from build123d import *

# Parameters (mm, degrees)
SKETCH1_R           = 2.75
BOSS_EXTRUDE1_DEPTH = 3
BOSS_EXTRUDE2_DEPTH = 3
CUT_EXTRUDE3_DEPTH  = 3.981121947


with BuildPart() as part:
    # Sketch1 → Boss-Extrude1 (new body)
    with BuildSketch(Plane(origin=(0, 0, 0), x_dir=(1, 0, 0), z_dir=(0, 1, 0))):
        with Locations(Location((0, 0, 0), (0, 0, 270))):
            Circle(SKETCH1_R)
    extrude(amount=BOSS_EXTRUDE1_DEPTH)

    # Sketch2 → Boss-Extrude2 (add)
    with BuildSketch(Plane(origin=(0, 0, 0), x_dir=(1, 0, 0), z_dir=(0, 1, 0))):
        Polygon((0.721687836, 1.25), (-0.721687836, 1.25), (-1.443375673, 0), (-0.721687836, -1.25), (0.721687836, -1.25), (1.443375673, 0), align=None)
    extrude(amount=BOSS_EXTRUDE2_DEPTH)

    # Sketch2_2 → Cut-Extrude3 (cut)
    with BuildSketch(Plane(origin=(0, 0, 0), x_dir=(1, 0, 0), z_dir=(0, 1, 0))):
        Polygon((0.721687836, 1.25), (-0.721687836, 1.25), (-1.443375673, 0), (-0.721687836, -1.25), (0.721687836, -1.25), (1.443375673, 0), align=None)
    extrude(amount=CUT_EXTRUDE3_DEPTH, mode=Mode.SUBTRACT)


solid = part.part
Build history of the part. All positions in model axes, mm. A direction names the side the tool comes from. Coordinates: 2 decimals unless noted, no trailing zeros. Order: outer loops, then holes, each group sorted by start corner. A loop starts at its lowest first (then second) coordinate and runs counter-clockwise, first axis right, second up. Notation, with made-up numbers: (66, 64) - (101, 64) arc R25 cw to (101, 93) - close; hole circle Ø3 at (14, 78). An arc over 180 degrees is marked (long way). Put each result on its own line as item: value.
1. Drop flat-ended pins along their axis: P1, Ø1.5, axis at y = 1.5, z = -1, coming from the -X side; P2, Ø1, axis at x = 1.5, z = 1.5, coming from the -Y side; P3, Ø0.7, axis at x = 0.5, y = 2, coming from the +Z side; P4, Ø1, axis at x = 2, y = 1.5, coming from the +Z side. Give the stop position or say it passes through.
Answer sheet:
P1: stops at x = -2.74
P2: stops at y = 0
P3: stops at z = 2.75
P4: stops at z = 2.3
2. Saw through at B-B (x = 0). Write the cut outline in (y, z).
Answer sheet:
outline: (0, -2.75) - (3, -2.75) - (3, -1.25) - (0, -1.25) - close; (0, 1.25) - (3, 1.25) - (3, 2.75) - (0, 2.75) - close
3. Saw through at A-A (y = 0.8). Write the cut outline in (x, z).
Answer sheet:
outline: circle Ø5.5 at (0, 0); hole (-1.44, 0) - (-0.72, -1.25) - (0.72, -1.25) - (1.44, 0) - (0.72, 1.25) - (-0.72, 1.25) - close
4. Probe line 1 along Z through (x, y) = (-0.05, 1.2); line 2 along Z through (x, y) = (1.3, 0.5); line 3 along Z through (x, y) = (2.45, 0.4). List the from-to ranges inside material, lowest first. Write a range as [from, to].
Answer sheet:
line 1: z = [-2.75, -1.25], [1.25, 2.75]
line 2: z = [-2.42, -0.25], [0.25, 2.42]
line 3: z = [-1.25, 1.25]
5. Saw through at C-C (z = 0.1). Write the cut outline in (x, y).
Answer sheet:
outline: (-2.75, 0) - (-1.39, 0) - (-1.39, 3) - (-2.75, 3) - close; (1.39, 0) - (2.75, 0) - (2.75, 3) - (1.39, 3) - close
6. Saw through at D-D (x = 1.75). Write the cut outline in (y, z), and give its area (3 significant figures).
Answer sheet:
outline: (0, -2.12) - (3, -2.12) - (3, 2.12) - (0, 2.12) - close
area: 12.7 mm^2
7. Tool access for faces 1 (the face through (1.3, 0, 0.6)), 2 (the face through (0, 1, 1.25)): list every direction of +Z, -Z, +X, -X, +Y, -Y with a clear straight run to the whole face (end or side of a thin tool).
Answer sheet:
face 1: +Z, -Z, +X, -X, -Y
face 2: +Y, -Y
8. Pull direction X, two halves, no side cores. Call faces 3 (the face through (-2.685, 1.479, -0.596)), 4 (the face through (1.3, 3, 0.6)), 5 (the face through (-1.08, 1.48, -0.63)): pulls with the +X half, pulls with the -X half, needs draft (parallel to the pull), parting line crosses it, or undercut.
Answer sheet:
face 3: parting line crosses it
face 4: needs draft
face 5: undercut
